Read the model definition and answer for the solid it produces. Units are mm, in the model's axes. A direction names the side the tool comes from. Give positions to 0.01 mm unless a question says otherwise; leave off trailing zeros. Order: outer loops, then holes, each group sorted by start corner. A loop starts at its lowest first (then second) coordinate and runs counter-clockwise, first axis right, second up. Notation, with made-up numbers: M -39,-7 L -16,-7 A12 cw -16,5 Z; hole C 53.25,21 d5. An arc over 180 degrees is marked long. One line per item, written item: value.
from build123d import *

# Parameters (mm, degrees)
SKETCH1_W           = 40
SKETCH1_H           = 20
BOSS_EXTRUDE2_DEPTH = 40
CUT_EXTRUDE1_DEPTH  = 40
BOSS_EXTRUDE3_DEPTH = 20
BOSS_EXTRUDE4_DEPTH = 20
CUT_EXTRUDE2_DEPTH  = 20
SKETCH6_W           = 20
SKETCH6_H           = 20
CUT_EXTRUDE3_DEPTH  = 109
BOSS_EXTRUDE5_DEPTH = 20
BOSS_EXTRUDE6_DEPTH = 20
CUT_EXTRUDE5_DEPTH  = 20


with BuildPart() as part:
    # Sketch1 → Boss-Extrude2 (new body)
    with BuildSketch(Plane.XY):
        with Locations((20, 10)):
            Rectangle(SKETCH1_W, SKETCH1_H)
    extrude(amount=BOSS_EXTRUDE2_DEPTH)

    # Sketch2 → Cut-Extrude1 (cut)
    with BuildSketch(Plane(origin=(0, 20, 0), x_dir=(1, 0, 0), z_dir=(0, 1, 0))):
        Polygon((0, -40), (20, 0), (0, 0), align=None)
    extrude(amount=-CUT_EXTRUDE1_DEPTH, mode=Mode.SUBTRACT)

    # Sketch3 → Boss-Extrude3 (add)
    with BuildSketch(Plane(origin=(0, 20, 0), x_dir=(1, 0, 0), z_dir=(0, 1, 0))):
        Polygon((40, -40), (40, 0), (20, -40), align=None)
    extrude(amount=BOSS_EXTRUDE3_DEPTH)

    # Sketch4 → Boss-Extrude4 (add)
    with BuildSketch(Plane(origin=(0, 20, 0), x_dir=(1, 0, 0), z_dir=(0, 1, 0))):
        Polygon((0, -40), (20, 0), (40, 0), (20, -40), align=None)
    extrude(amount=BOSS_EXTRUDE4_DEPTH)

    # Sketch5 → Cut-Extrude2 (cut)
    with BuildSketch(Plane(origin=(0, 40, 0), x_dir=(1, 0, 0), z_dir=(0, 1, 0))):
        Polygon((40, 0), (20, -40), (40, -40), align=None)
    extrude(amount=-CUT_EXTRUDE2_DEPTH, mode=Mode.SUBTRACT)

    # Sketch6 → Cut-Extrude3 (cut)
    with BuildSketch(Plane.XY.offset(40)):
        with Locations((10, 30)):
            Rectangle(SKETCH6_W, SKETCH6_H)
    extrude(amount=-CUT_EXTRUDE3_DEPTH, mode=Mode.SUBTRACT)

    # Sketch7 → Boss-Extrude5 (add)
    with BuildSketch(Plane(origin=(0, 20, 0), x_dir=(1, 0, 0), z_dir=(0, 1, 0))):
        Polygon((20, 0), (0, 0), (0, -40), align=None)
    extrude(amount=-BOSS_EXTRUDE5_DEPTH)

    # Sketch8 → Boss-Extrude6 (add)
    with BuildSketch(Plane(origin=(0, 20, 0), x_dir=(1, 0, 0), z_dir=(0, 1, 0))):
        Polygon((20, -40), (40, -40), (40, 0), align=None)
    extrude(amount=BOSS_EXTRUDE6_DEPTH)

    # Sketch9 → Cut-Extrude5 (cut)
    with BuildSketch(Plane(origin=(0, 40, 0), x_dir=(1, 0, 0), z_dir=(0, 1, 0))):
        Polygon((20, -40), (30, -20), (20, 0), align=None)
        Polygon((40, -40), (30, -20), (20, -40), align=None)
    extrude(amount=-CUT_EXTRUDE5_DEPTH, mode=Mode.SUBTRACT)


solid = part.part
1) Consider probe 1 along Y at (x, z) = (18, 26); probe 2 along X at (y, z) = (36, 2); probe 3 along X at (y, z) = (30.5, 30.5). Determine where each line is inside the solid, lowest interval first.
Reported:
probe 1: y = 0 to 20
probe 2: x = 21 to 40
probe 3: x = 35.25 to 40
2) Find section B-B, the plane z = 28.5. Write down the section's boundary in (x, y), plus the area to 3 significant figures.
Reported:
outline: M 0,0 L 40,0 L 40,40 L 34.25,40 L 34.25,20 L 0,20 Z
area: 915 mm^2
3) Find section A-A, the plane x = 23. Write down the section's boundary in (y, z), plus the area to 3 significant figures.
Reported:
outline: M 0,0 L 40,0 L 40,6 L 20,6 L 20,40 L 0,40 Z
area: 920 mm^2
4) This flat-tipped pin is pushed along its axis until it touches: pin 1 Ø5 at (x, z) = (26, 31) entering from +Y. Where does it stop, or does it pass through?
Reported:
pin 1: stops at y = 20
5) Find section D-D, the plane x = 18.5. Write down the section's boundary in (y, z), plus the area to 3 significant figures.
Reported:
outline: M 0,0 L 20,0 L 20,40 L 0,40 Z
area: 800 mm^2
6) Which of the six approach directions +Z, -Z, +X, -X, +Y, -Y give full straight-line access (tool end or side, diameter ignored) to faces 1 (the face through (34, 40, 11)), 2 (the face through (30, 30, 20))?
Reported:
face 1: +Z, -Z, +X, -X, +Y
face 2: +Z, -X, +Y
7) Find section C-C, the plane y = 33. Write down the section's boundary in (x, z), plus the area to 3 significant figures.
Reported:
outline: M 20,0 L 40,0 L 40,40 Z
area: 400 mm^2
